Geometry check sheet. Reference: the model listing, model coordinates, mm. Round coordinates to 2 decimals unless told otherwise and drop trailing zeros. Write each loop counter-clockwise with the first axis right and the second up, starting at its lowest first coordinate (ties: lowest second). Pieces come first, ordered by that corner, then holes.
Item 1: Depth check by flat-ended pin: P1, Ø1, axis at x = -7, z = 25.5, coming from the -Y side. Enter the tip coordinate at first touch or a pass-through.
Item 2: Cross-section at D-D (x = -1.75). Enter the section's corners in (y, z).
Item 3: Cross-section at A-A (y = 10). Enter the section's corners in (x, z), then the cut area to 3 significant figures.
Item 4: Draft check along X on faces 1 (the face through (-5, 12, 26)), 2 (the face through (-2.8, 10.1, 25)), 3 (the face through (0, 10, 26)). Enter one of: pulls with the +X half, pulls with the -X half, needs draft (parallel to the pull), parting line crosses it, or undercut.
Item 5: Cross-section at C-C (z = 26.7). Enter the section's corners in (x, y).
Item 6: Scan lines: probe 1 along Y at (x, z) = (-3.5, 26); probe 2 along Y at (x, z) = (-5, 26); probe 3 along X at (y, z) = (11.5, 26.2). Record each from-to range of solid material in increasing order.
Item 7: Cross-section at B-B (x = -3.25). Enter the section's corners in (y, z).
from build123d import *

# Parameters (mm, degrees)
BOX010_W          = 10
BOX010_H          = 20
BOX010_DEPTH      = 2.5
CYLINDER004_R     = 2
CYLINDER004_DEPTH = 2.5
CYLINDER005_R     = 10
CYLINDER005_DEPTH = 2.5


with BuildPart() as cubo002:
    # Box010 → Box010 (new body)
    with BuildSketch(Plane.XY.offset(25)):
        with Locations((5, 10)):
            Rectangle(BOX010_W, BOX010_H)
    extrude(amount=BOX010_DEPTH)


with BuildPart() as cilindro004:
    # Cylinder004 → Cylinder004 (new body)
    with BuildSketch(Plane(origin=(-5, 10, 25), x_dir=(1, 0, 0), z_dir=(0, 0, 1))):
        Circle(CYLINDER004_R)
    extrude(amount=CYLINDER004_DEPTH)


with BuildPart() as cut010:
    # Cylinder005 → Cylinder005 (new body)
    with BuildSketch(Plane(origin=(0, 10, 25), x_dir=(1, 0, 0), z_dir=(0, 0, 1))):
        Circle(CYLINDER005_R)
    extrude(amount=CYLINDER005_DEPTH)

    # Cut009: cut Cilindro004
    add(cilindro004.part, mode=Mode.SUBTRACT)

    # Cut010: cut Cubo002
    add(cubo002.part, mode=Mode.SUBTRACT)


solid = cut010.part
Resolved:
1. P1: stops at y = 2.4
2. outline: (0.15, 25) - (19.85, 25) - (19.85, 27.5) - (0.15, 27.5) - close
3. outline: (-10, 25) - (-7, 25) - (-7, 27.5) - (-10, 27.5) - close; (-3, 25) - (0, 25) - (0, 27.5) - (-3, 27.5) - close
3. area: 15.0 mm2
4. face 1: undercut
4. face 2: needs draft
4. face 3: pulls with the +X half
5. outline: (0, 0) - (0, 20) arc R10 ccw to start; hole circle Ø4 at (-5, 10)
6. probe 1: y = 0.63 to 8.68, 11.32 to 19.37
6. probe 2: y = 1.34 to 8, 12 to 18.66
6. probe 3: x = -9.89 to -6.32, -3.68 to 0
7. outline: (0.54, 25) - (9.03, 25) - (9.03, 27.5) - (0.54, 27.5) - close; (10.97, 25) - (19.46, 25) - (19.46, 27.5) - (10.97, 27.5) - close
